Read the model definition and answer for the solid it produces. Units are mm, in the model's axes. A direction names the side the tool comes from. Coordinates: 2 decimals unless noted, no trailing zeros. Write each loop counter-clockwise with the first axis right and the second up, starting at its lowest first coordinate (ties: lowest second). Pieces come first, ordered by that corner, then holes. Notation, with made-up numbers: (64, 77) -> (83, 77) arc R29 ccw to (83, 99) -> close; hole circle Ø3 at (32.5, 88.25). An arc over 180 degrees is marked (long way). Answer as a JSON object with one key per item and string values. Group by question number.
(1) For a pull along X with two mould halves and no side action, classify faces 3 (the face through (5.5, 123, 6)), 4 (the face through (-10, 123, 0)), 5 (the face through (-7, 123, -10)), 6 (the face through (0, 123, 3.9)) as +X half, -X half, draft (parallel to the pull), parting line (faces both ways), or undercut.
(2) Straight lines are drawn through the part: L1, parallel to Z at x = 3.5, y = 172.5; L2, parallel to X at y = 97, z = -6; L3, parallel to X at y = 128.5, z = 8.25 (3 decimals). For each, find the intervals that lie inside material, in ascending order.
(3) Find section A-A (y = 22.5). Give the vertices of the cut face in (x, z) (3 decimals).
(4) Which of the six approach directions +Z, -Z, +X, -X, +Y, -Y give full straight-line access (tool end or side, diameter ignored) to faces 1 (the face through (10, 123, 0)), 2 (the face through (-5.5, 123, -6))?
(5) A flat-ended cylindrical pin translates along its axis: P1, Ø3, axis at x = 1, z = -6.5, coming from the +Y side. Find the tip coordinate at first contact, or state that the pin passes through.
Autodesk Inventor part; units mm, degrees
ref_plane "YZ Plane" through (0, 0, 0) normal (1, 0, 0) x (0, 1, 0)
ref_plane "XZ Plane" through (0, 0, 0) normal (0, 1, 0) x (-1, 0, 0)
ref_plane "XY Plane" through (0, 0, 0) normal (0, 0, 1) x (1, 0, 0)
sketch "Sketch1" plane through (0, 0, 0) normal (0, 1, 0) x (-1, 0, 0)
  line L0 (10, 10) -> (10, -10)
  line L1 (-10, -10) -> (-10, 10)
  line L2 (3.125, -10) -> (3.125, -8.2)
  line L3 (3.125, -8.2) -> (5.5, -8.2)
  line L4 (5.5, -8.2) -> (5.5, -3.9)
  line L5 (5.5, -3.9) -> (-5.5, -3.9)
  line L6 (-5.5, -3.9) -> (-5.5, -8.2)
  line L7 (-5.5, -8.2) -> (-3.125, -8.2)
  line L8 (-3.125, -8.2) -> (-3.125, -10)
  line L9 (10, -10) -> (3.125, -10)
  line L10 (-3.125, -10) -> (-10, -10)
  line L11 (3.125, 10) -> (3.125, 8.2)
  line L12 (3.125, 8.2) -> (5.5, 8.2)
  line L13 (5.5, 8.2) -> (5.5, 3.9)
  line L14 (5.5, 3.9) -> (-5.5, 3.9)
  line L15 (-5.5, 3.9) -> (-5.5, 8.2)
  line L16 (-5.5, 8.2) -> (-3.125, 8.2)
  line L17 (-3.125, 8.2) -> (-3.125, 10)
  line L18 (-10, 10) -> (-3.125, 10)
  line L19 (3.125, 10) -> (10, 10)
  point P0 (0, 0)
  dimension "d0" = 20
  dimension "d1" = 20
  dimension "d4" = 2.375
  dimension "d5" = 4.3
  dimension "d6" = 11
  dimension "d7" = 2.375
  dimension "d8" = 1.8
  dimension "d9" = 6.875
  dimension "d10" = 1.8
  dimension "d11" = 4.3
extrude "Extrusion1" add sketch "Sketch1" along normal blind 250
properties part number "Perfil"
Results below:
{
 "1": {"face 3": "undercut", "face 4": "-X half", "face 5": "draft", "face 6": "undercut"},
 "2": {"L1": "z = -10 to -8.2, -3.9 to 3.9, 8.2 to 10", "L2": "x = -10 to -5.5, 5.5 to 10", "L3": "x = -10 to -3.125, 3.125 to 10"},
 "3": {"outline": "(-10, -10) -> (-3.125, -10) -> (-3.125, -8.2) -> (-5.5, -8.2) -> (-5.5, -3.9) -> (5.5, -3.9) -> (5.5, -8.2) -> (3.125, -8.2) -> (3.125, -10) -> (10, -10) -> (10, 10) -> (3.125, 10) -> (3.125, 8.2) -> (5.5, 8.2) -> (5.5, 3.9) -> (-5.5, 3.9) -> (-5.5, 8.2) -> (-3.125, 8.2) -> (-3.125, 10) -> (-10, 10) -> close"},
 "4": {"face 1": "+Z, -Z, +X, +Y, -Y", "face 2": "+Y, -Y"},
 "5": {"P1": "passes through"}
}
